The model under review builds one solid part; all positions refer to its coordinate system, in mm. A direction names the side the tool comes from. Round coordinates to 2 decimals unless told otherwise and drop trailing zeros. Write each loop counter-clockwise with the first axis right and the second up, starting at its lowest first coordinate (ties: lowest second). Pieces come first, ordered by that corner, then holes. Notation, with made-up numbers: (23, -1.75) - (67, -1.75) arc R16 cw to (67, 24.25) - close; hole circle Ø10 at (-17, -19.5). An arc over 180 degrees is marked (long way). Use one line per item in the form item = value.
Autodesk Inventor part; units mm, degrees
ref_plane "YZ Plane" through (0, 0, 0) normal (1, 0, 0) x (0, 1, 0)
ref_plane "XZ Plane" through (0, 0, 0) normal (0, 1, 0) x (-1, 0, 0)
ref_plane "XY Plane" through (0, 0, 0) normal (0, 0, 1) x (1, 0, 0)
sketch "Sketch1" plane through (0, 0, 0) normal (0, 0, 1) x (1, 0, 0)
  line L0 (-18.8022, 16.0864) -> (131.1978, 16.0864)
  line L1 (131.1978, 16.0864) -> (131.1978, -133.9136)
  line L2 (131.1978, -133.9136) -> (-18.8022, -133.9136)
  line L3 (-18.8022, -133.9136) -> (-18.8022, 16.0864)
  point P0 (0, 0)
  dimension "d0" = 150
  dimension "d1" = 150
extrude "Extrusion1" add sketch "Sketch1" along normal blind 35
sketch "Sketch2" plane through (0, 0, 35) normal (0, 0, 1) x (1, 0, 0)
  line L0 (-18.8022, -133.9136) -> (131.1978, -133.9136)
  line L1 (-18.8022, 16.0864) -> (-18.8022, -133.9136)
  line L2 (131.1978, -133.9136) -> (131.1978, 16.0864)
  line L3 (-18.8022, 16.0864) -> (1.1978, 16.0864)
  line L4 (131.1978, 16.0864) -> (-18.8022, 16.0864)
  line L5 (131.1978, 16.0864) -> (111.1978, 16.0864)
  arc A0 (1.1978, 16.0864) -> (111.1978, 16.0864) centre (56.1978, 40.0655) ccw
  line L6 (1.1978, 16.0864) -> (111.1978, 16.0864)
  line L7 (56.1978, -93.9136) -> (-18.8022, -93.9136)
  line L8 (56.1978, -93.9136) -> (131.1978, -93.9136)
  line L9 (56.1978, -93.9136) -> (11.1978, -93.9136)
  line L10 (11.1978, -93.9136) -> (11.1978, -33.9136)
  line L11 (11.1978, -33.9136) -> (101.1978, -33.9136)
  line L12 (101.1978, -33.9136) -> (101.1978, -93.9136)
  point P0 (0, 0)
  dimension "d5" = 20
  dimension "d6" = 20
  dimension "d7" = 60
  dimension "d10" = 60
  dimension "d11" = 90
  dimension "d12" = 60
extrude "Extrusion2" cut sketch "Sketch2" against normal blind 35 contours L4 A0
extrude "Extrusion3" cut sketch "Sketch2" against normal blind 15 contours L10 L11 L12 L8 L7
properties part number "Version1"
(1) Add section A-A on z = 25. Write out the cut boundary in (x, y), then the cut area to 3 significant figures.
Geometry results:
outline = (-18.8, -133.91) - (131.2, -133.91) - (131.2, 16.09) - (111.2, 16.09) arc R60 cw to (1.2, 16.09) - (-18.8, 16.09) - close; hole (11.2, -93.91) - (101.2, -93.91) - (101.2, -33.91) - (11.2, -33.91) - close
area = 14,200 mm2
(2) Add section B-B on x = 39. Write out the cut boundary in (y, z).
Geometry results:
outline = (-133.91, 0) - (-17.42, 0) - (-17.42, 35) - (-33.91, 35) - (-33.91, 20) - (-93.91, 20) - (-93.91, 35) - (-133.91, 35) - close
(3) To check wall thickness, follow L1, parallel to X at y = -61.5, z = 31; L2, parallel to Y at x = 14.5, z = 23; L3, parallel to Z at x = 16.5, y = -54.5. State the ranges of each line that lie inside material, in increasing order.
Geometry results:
L1 = -18.8 to 11.2, 101.2 to 131.2
L2 = -133.91 to -93.91, -33.91 to -3.08
L3 = 0 to 20
(4) Add section C-C on y = -66. Write out the cut boundary in (x, z), then the cut area to 3 significant figures.
Geometry results:
outline = (-18.8, 0) - (131.2, 0) - (131.2, 35) - (101.2, 35) - (101.2, 20) - (11.2, 20) - (11.2, 35) - (-18.8, 35) - close
area = 3,900 mm2
(5) Insertion check: P1, Ø5, axis at x = 5.5, z = 9, coming from the +Y side; P2, Ø16.5, axis at x = 36, z = 24, coming from the +Y side. Each pin has a flat end and moves straight along its axis. Give the tip position at first contact, or say it passes through.
Geometry results:
P1 = 12.32
P2 = -12.76
(6) Add section D-D on z = 5. Write out the cut boundary in (x, y).
Geometry results:
outline = (-18.8, -133.91) - (131.2, -133.91) - (131.2, 16.09) - (111.2, 16.09) arc R60 cw to (1.2, 16.09) - (-18.8, 16.09) - close
(7) The part is to be moulded in two halves that separate along X. For faces 3 (the cylindrical face through (55.224, -19.927, 17.745)), 4 (the flat face through (121, 16.086, 17)), 5 (the flat face through (131.198, -58, 17)), say which applies: +X half, -X half, draft (parallel to the pull), parting line (faces both ways), or undercut.
Geometry results:
face_3 = undercut
face_4 = draft
face_5 = +X half
(8) Machinability: for faces 1 (the flat face through (101.198, -63, 28)), 2 (the flat face through (55, -75, 0)), which of the approach directions +Z, -Z, +X, -X, +Y, -Y give a long, thin tool a straight path to every point of the face, cutting with its end or side? Answer none if there is none.
Geometry results:
face_1 = +Z
face_2 = -Z, +X, -X, +Y, -Y
